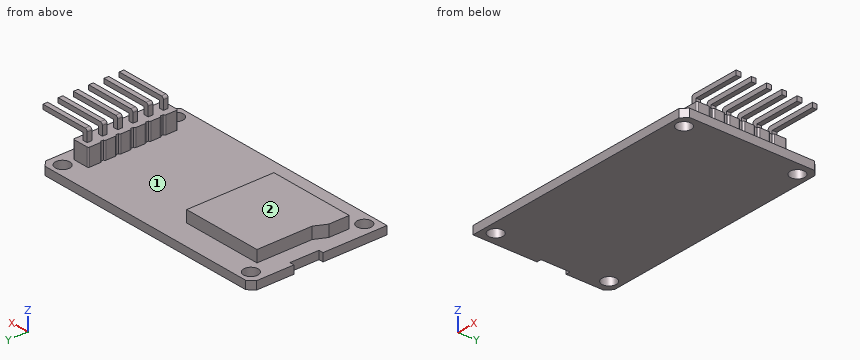
from build123d import *

# Parameters (mm, degrees)
BOSS_EXTRUDE1_DEPTH        = 1.4
F_2_5_2_5_DIAMETER_SLOT1_D = 2.5
BOSS_EXTRUDE2_DEPTH        = 2
BOSS_EXTRUDE3_DEPTH        = 3
SKETCH8_W                  = 0.8
SKETCH8_H                  = 0.8
BOSS_EXTRUDE4_DEPTH        = 2
SKETCH9_W                  = 0.8
SKETCH9_H                  = 0.8
BOSS_EXTRUDE5_DEPTH        = 8
LPATTERN1_COUNT            = 6
LPATTERN1_PITCH            = 2.62
FILLET1_R                  = 0.4


with BuildPart() as part:
    # Sketch1 → Boss-Extrude1 (new body)
    with BuildSketch(Plane.XY):
        Polygon((-17.623529412, 11.42), (-16.623529412, 12.42), (23.376470588, 12.42), (24.376470588, 11.42), (24.376470588, -10), (23.376470588, -11), (-17.623529412, -11), (-17.623529412, 0), (-16.823529412, 0), (-16.823529412, 5), (-17.623529412, 5), align=None)
    extrude(amount=BOSS_EXTRUDE1_DEPTH)

    # Ø2.5 (2.5) Diameter Slot1 (through all)
    with Locations(Plane.XY.offset(1.4)):
        with Locations((-15.373529412, -9.04), (-15.373529412, 10.46), (22.126470588, -9.04), (22.126470588, 10.46)):
            Hole(F_2_5_2_5_DIAMETER_SLOT1_D / 2)

    # Sketch6 → Boss-Extrude2 (add)
    with BuildSketch(Plane.XY.offset(1.4)):
        Polygon((-15.083529412, -6.7), (-0.083529412, -6.7), (-0.083529412, 8.3), (-14.083529412, 8.3), (-14.083529412, -1.2), (-15.083529412, -3.2), align=None)
    extrude(amount=BOSS_EXTRUDE2_DEPTH)

    # Sketch7 → Boss-Extrude3 (add)
    with BuildSketch(Plane.XY.offset(1.4)):
        with BuildLine():
            Line((22.126470588, 6.1), (22.126470588, 5.6))
            ThreePointArc((22.126470588, 5.6), (22.303247284, 5.526776695), (22.376470588, 5.35))
            Line((22.376470588, 5.35), (22.376470588, 3.78))
            ThreePointArc((22.376470588, 3.78), (22.303247284, 3.603223305), (22.126470588, 3.53))
            Line((22.126470588, 3.53), (22.126470588, 3.03))
            ThreePointArc((22.126470588, 3.03), (22.303247284, 2.956776695), (22.376470588, 2.78))
            Line((22.376470588, 2.78), (22.376470588, 1.21))
            ThreePointArc((22.376470588, 1.21), (22.303247284, 1.033223305), (22.126470588, 0.96))
            Line((22.126470588, 0.96), (22.126470588, 0.46))
            ThreePointArc((22.126470588, 0.46), (22.303247284, 0.386776695), (22.376470588, 0.21))
            Line((22.376470588, 0.21), (22.376470588, -1.36))
            ThreePointArc((22.376470588, -1.36), (22.303247284, -1.536776695), (22.126470588, -1.61))
            Line((22.126470588, -1.61), (22.126470588, -2.11))
            ThreePointArc((22.126470588, -2.11), (22.303247284, -2.183223305), (22.376470588, -2.36))
            Line((22.376470588, -2.36), (22.376470588, -3.93))
            ThreePointArc((22.376470588, -3.93), (22.303247284, -4.106776695), (22.126470588, -4.18))
            Line((22.126470588, -4.18), (22.126470588, -4.68))
            ThreePointArc((22.126470588, -4.68), (22.303247284, -4.753223305), (22.376470588, -4.93))
            Line((22.376470588, -4.93), (22.376470588, -6.75))
            ThreePointArc((22.376470588, -6.75), (22.303247284, -6.926776695), (22.126470588, -7))
            Line((22.126470588, -7), (19.626470588, -7))
            ThreePointArc((19.626470588, -7), (19.449693893, -6.926776695), (19.376470588, -6.75))
            Line((19.376470588, -6.75), (19.376470588, -4.93))
            ThreePointArc((19.376470588, -4.93), (19.449693893, -4.753223305), (19.626470588, -4.68))
            Line((19.626470588, -4.68), (19.626470588, -4.18))
            ThreePointArc((19.626470588, -4.18), (19.449693893, -4.106776695), (19.376470588, -3.93))
            Line((19.376470588, -3.93), (19.376470588, -2.36))
            ThreePointArc((19.376470588, -2.36), (19.449693893, -2.183223305), (19.626470588, -2.11))
            Line((19.626470588, -2.11), (19.626470588, -1.61))
            ThreePointArc((19.626470588, -1.61), (19.449693893, -1.536776695), (19.376470588, -1.36))
            Line((19.376470588, -1.36), (19.376470588, 0.21))
            ThreePointArc((19.376470588, 0.21), (19.449693893, 0.386776695), (19.626470588, 0.46))
            Line((19.626470588, 0.46), (19.626470588, 0.96))
            ThreePointArc((19.626470588, 0.96), (19.449693893, 1.033223305), (19.376470588, 1.21))
            Line((19.376470588, 1.21), (19.376470588, 2.78))
            ThreePointArc((19.376470588, 2.78), (19.449693893, 2.956776695), (19.626470588, 3.03))
            Line((19.626470588, 3.03), (19.626470588, 3.53))
            ThreePointArc((19.626470588, 3.53), (19.449693893, 3.603223305), (19.376470588, 3.78))
            Line((19.376470588, 3.78), (19.376470588, 5.35))
            ThreePointArc((19.376470588, 5.35), (19.449693893, 5.526776695), (19.626470588, 5.6))
            Line((19.626470588, 5.6), (19.626470588, 6.1))
            ThreePointArc((19.626470588, 6.1), (19.449693893, 6.173223305), (19.376470588, 6.35))
            Line((19.376470588, 6.35), (19.376470588, 8.17))
            ThreePointArc((19.376470588, 8.17), (19.449693893, 8.346776695), (19.626470588, 8.42))
            Line((19.626470588, 8.42), (22.126470588, 8.42))
            ThreePointArc((22.126470588, 8.42), (22.303247284, 8.346776695), (22.376470588, 8.17))
            Line((22.376470588, 8.17), (22.376470588, 6.35))
            ThreePointArc((22.376470588, 6.35), (22.303247284, 6.173223305), (22.126470588, 6.1))
        make_face()
    extrude(amount=BOSS_EXTRUDE3_DEPTH)

    # Sketch8 → Boss-Extrude4 (add)
    with BuildSketch(Plane.XY.offset(4.4)):
        with Locations((20.876470588, -5.84)):
            Rectangle(SKETCH8_W, SKETCH8_H)
        with Locations((20.876470588, -3.22)):
            Rectangle(SKETCH8_W, SKETCH8_H)
        with Locations((20.876470588, -0.6)):
            Rectangle(SKETCH8_W, SKETCH8_H)
        with Locations((20.876470588, 2.02)):
            Rectangle(SKETCH8_W, SKETCH8_H)
        with Locations((20.876470588, 4.64)):
            Rectangle(SKETCH8_W, SKETCH8_H)
        with Locations((20.876470588, 7.26)):
            Rectangle(SKETCH8_W, SKETCH8_H)
    extrude(amount=BOSS_EXTRUDE4_DEPTH)

    # Sketch9 → Boss-Extrude5 (add)
    with BuildSketch(Plane(origin=(21.276470588, 0, 0), x_dir=(0, 0, -1), z_dir=(1, 0, 0))):
        with Locations((-6, 7.26)):
            Rectangle(SKETCH9_W, SKETCH9_H)
    boss_extrude5 = extrude(amount=BOSS_EXTRUDE5_DEPTH)

    # LPattern1: Boss-Extrude5 ×6
    with Locations(*[(0, -i * LPATTERN1_PITCH, 0) for i in range(1, LPATTERN1_COUNT)]):
        add(boss_extrude5)

    # Fillet1
    fillet1_edges = [part.edges().sort_by_distance(p)[0] for p in [
        (20.476470588, -5.84, 6.4),
        (20.476470588, -3.22, 6.4),
        (20.476470588, -0.6, 6.4),
        (20.476470588, 2.02, 6.4),
        (20.476470588, 4.64, 6.4),
        (20.476470588, 7.26, 6.4),
    ]]
    fillet(fillet1_edges, radius=FILLET1_R)


solid = part.part
Model file for the job. Use its own axes, mm. Face numbers are marked on the shaded views. Give positions to 0.01 mm unless a question says otherwise; leave off trailing zeros. Order: outer loops, then holes, each group sorted by start corner. A loop starts at its lowest first (then second) coordinate and runs counter-clockwise, first axis right, second up. Notation, with made-up numbers: (78.5, 83.25) -> (118.5, 83.25) arc R20 ccw to (118.5, 121.25) -> close; hole circle Ø8 at (7.25, 12.5). An arc over 180 degrees is marked (long way). Use CSV: the item, a comma, the result in double quotes.
1. Mould opens along X. For the marked faces 1 and 2 say: +X half, -X half, draft (parallel to the pull), parting line (faces both ways), or undercut.
Outcome:
face 1,"undercut"
face 2,"draft"
2. Band-saw the part on B-B, the plane x = -6. Give the cut face in (y, z).
Outcome:
outline,"(-11, 0) -> (12.42, 0) -> (12.42, 1.4) -> (8.3, 1.4) -> (8.3, 3.4) -> (-6.7, 3.4) -> (-6.7, 1.4) -> (-11, 1.4) -> close"
3. Band-saw the part on A-A, the plane y = 10.46. Give the cut face in (x, z), then the cut area to 3 significant figures.
Outcome:
outline,"(-17.62, 0) -> (-16.62, 0) -> (-16.62, 1.4) -> (-17.62, 1.4) -> close; (-14.12, 0) -> (20.88, 0) -> (20.88, 1.4) -> (-14.12, 1.4) -> close; (23.38, 0) -> (24.38, 0) -> (24.38, 1.4) -> (23.38, 1.4) -> close"
area,"51.8 mm²"
4. Band-saw the part on C-C, the plane x = 13.5. Give the cut face in (y, z), then the cut area to 3 significant figures.
Outcome:
outline,"(-11, 0) -> (12.42, 0) -> (12.42, 1.4) -> (-11, 1.4) -> close"
area,"32.8 mm²"
5. Drop flat-ended pins along their axis: pin 1 (1.5 mm diameter, centred on x = -6, y = 9, fed in from +Z); pin 2 (3 mm diameter, centred on x = 10, y = -3.5, fed in from +Z); pin 3 (0.6 mm diameter, centred on y = 1, z = 3, fed in from +X); pin 4 (1.5 mm diameter, centred on x = 22.13, y = 10.46, fed in from +Z) (3 decimals). Give the stop position or say it passes through.
Outcome:
pin 1,"z = 3.4"
pin 2,"z = 1.4"
pin 3,"x = 22.38"
pin 4,"through"
6. Drill centre lines: line 1 along X through (y, z) = (4.25, 3); line 2 along Z through (x, y) = (7, -8.75); line 3 along Y through (x, z) = (20, 2.5). Where is each one in solid material? Low to high. Write a range as from..to.
Outcome:
line 1,"-14.08..-0.08, 19.38..22.38"
line 2,"0..1.4"
line 3,"-7..8.42"
